Geometry: final body of the model. Coordinates: model frame, mm. Give positions to 0.01 mm unless a question says otherwise; leave off trailing zeros. Write each loop counter-clockwise with the first axis right and the second up, starting at its lowest first coordinate (ties: lowest second). Pieces come first, ordered by that corner, then holes. Notation, with made-up numbers: M 45,36.25 L 69,36.25 A35 ccw 69,70.25 Z; hole C 89.25,78 d10. An arc over 180 degrees is marked long. Use one line per item in the form item = value. Start each with the question number.
Item 1: Section query B-B on x = 15.5. Return loops of the section in (y, z), then the cut area to 3 significant figures.
Item 2: Material intervals for line 1 along Y through (x, z) = (-9, 65); line 2 along Z through (x, y) = (-13, 3); line 3 along X through (y, z) = (7, 37.5), sorted ascending. Write a range as from..to.
Item 3: Section query D-D on z = -2. Return loops of the section in (x, y).
Item 4: Section query A-A on y = 1.75. Return loops of the section in (x, z), then the cut area to 3 significant figures.
Item 5: Contact query for a flat-ended pin moving along its axis: P1, Ø1.5, axis at x = -33.5, z = -13, coming from the +Y side. Output: stop coordinate, or through.
Item 6: Section query C-C on z = 82.5. Return loops of the section in (x, y), then the cut area to 3 significant figures.
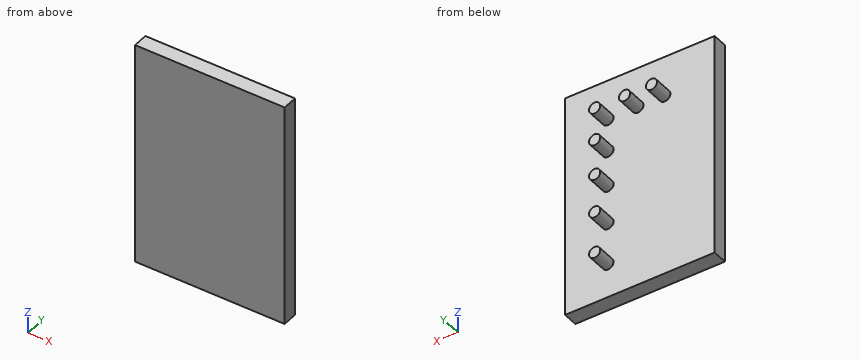
from build123d import *

# Parameters (mm, degrees)
F0_W     = 100
F0_H     = 150
F1_DEPTH = 10
F2_R     = 3.75
F3_DEPTH = 13


# Not quite as in the source:
# - a feature names something its author has since deleted; it is built from what else it names


with BuildPart() as f1:
    # F0 (on Front) → F1 (new body)
    with BuildSketch(Plane.XZ):
        with Locations((3.0784979463, 33.0328063236)):
            Rectangle(F0_W, F0_H)
    extrude(amount=F1_DEPTH)

    # F2 (on face) → F3 (join)
    with BuildSketch(Plane(origin=(0, 0, 0), x_dir=(-1, 0, 0), z_dir=(0, 1, 0))):
        with Locations((13.6121616811, 80.8424673975)):
            Circle(F2_R)
        with Locations((-4.3878383189, 80.8424673975)):
            Circle(F2_R)
        with Locations((-24.3878383189, 80.8424673975)):
            Circle(F2_R)
        with Locations((-24.3878383189, 58.8424673975)):
            Circle(F2_R)
        with Locations((-24.3878383189, 34.8424673975)):
            Circle(F2_R)
        with Locations((-24.3878383189, 8.8424673975)):
            Circle(F2_R)
        with Locations((-24.3878383189, -19.1575326025)):
            Circle(F2_R)
    extrude(amount=F3_DEPTH)


solid = f1.part
Answer sheet:
q1.outline = M -10,-41.97 L 0,-41.97 L 0,108.03 L -10,108.03 Z
q1.area = 1,500 mm2
q2.line_1 = -10..0
q2.line_2 = 77.14..84.54
q2.line_3 = 21.74..27.03
q3.outline = M -46.92,-10 L 53.08,-10 L 53.08,0 L -46.92,0 Z
q4.outline = C -13.61,80.84 d7.5; C 4.39,80.84 d7.5; C 24.39,-19.16 d7.5; C 24.39,8.84 d7.5; C 24.39,34.84 d7.5; C 24.39,58.84 d7.5; C 24.39,80.84 d7.5
q4.area = 309 mm2
q5.P1 = 0
q6.outline = M -46.92,-10 L 53.08,-10 L 53.08,0 L 27.75,0 L 27.75,13 L 21.02,13 L 21.02,0 L 7.75,0 L 7.75,13 L 1.02,13 L 1.02,0 L -10.25,0 L -10.25,13 L -16.98,13 L -16.98,0 L -46.92,0 Z
q6.area = 1,260 mm2
